Answer from the drawing. Dimensions are ordinates in mm from the lowest x, y and z of the part. A direction names the side the tool comes from. Round coordinates to 2 decimals unless told otherwise and drop trailing zeros. Write each loop counter-clockwise with the first axis right and the second up, starting at its lowest first coordinate (ties: lowest second). Pieces come first, ordered by that corner, then holes. Notation, with made-up numbers: (64.25, 26.5) -> (101.25, 26.5) arc R18 ccw to (101.25, 48.5) -> close; hole circle Ø1 at (45.25, -37.5). An arc over 180 degrees is marked (long way). Answer as a JSON object with one key per item and string values. Group by question number.
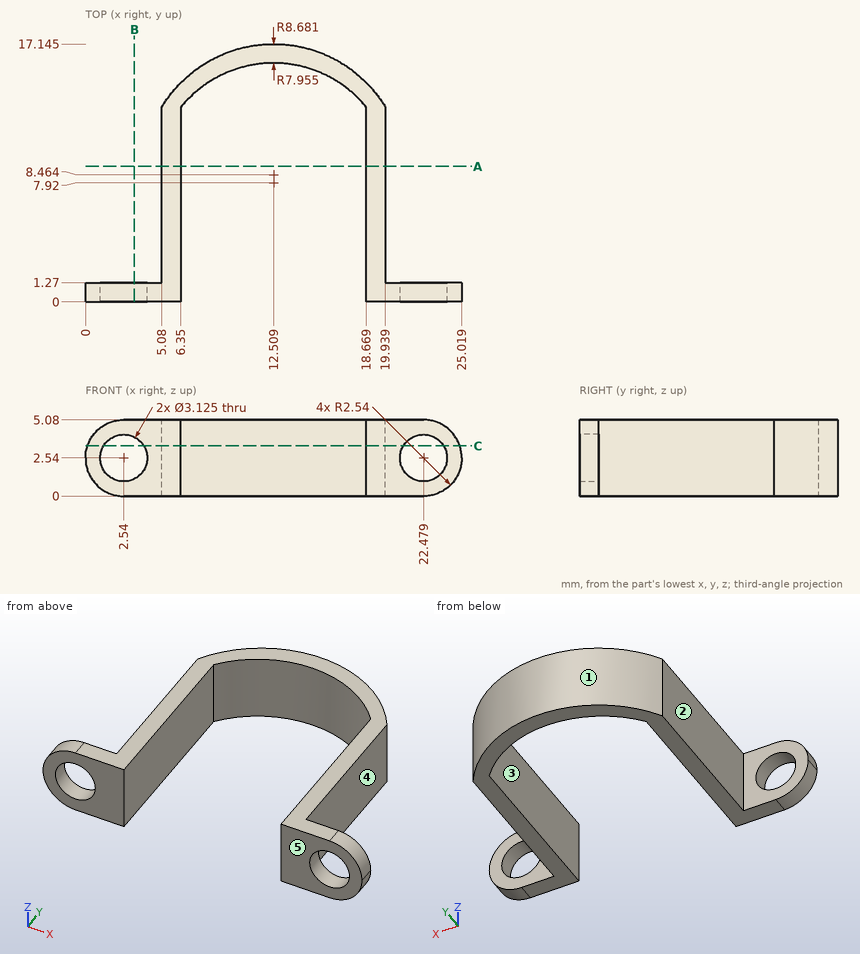
1) A cutting plane is placed at A-A on y = 9. Determine the outline of the cut face in (x, z).
2) A cutting plane is placed at B-B on x = 3.25. Determine the outline of the cut face in (y, z).
3) Each of these flat-tipped pins is pushed along its axis until it touches: P1, Ø3, axis at y = 10.5, z = 4.5, coming from the +X side; P2, Ø2.5, axis at x = 2.5, z = 3, coming from the +Y side; P3, Ø10, axis at x = 9, y = 5.5, coming from the +Z side; P4, Ø2, axis at x = 17, y = 8.5, coming from the +Z side. Where does it stop, or does it pass through?
4) Straight lines are drawn through the part: L1, parallel to X at y = 0.3, z = 2.54; L2, parallel to X at y = 4, z = 0.3; L3, parallel to Y at x = 24.25, z = 2.4. For each, find the intervals that lie inside material, in ascending order.
5) A tool of negligible diameter and unlimited length cuts with its end or side. For the marked faces 1, 2, 3, 4 and 5, from which of +Z, -Z, +X, -X, +Y, -Y can it reach the whole face along a straight path? Write none if from no direction.
6) A cutting plane is placed at C-C on z = 3.35. State how many separate pieces and enclosed holes the cut face has.
Established:
{
 "1": {"outline": "(5.08, 0) -> (6.35, 0) -> (6.35, 5.08) -> (5.08, 5.08) -> close; (18.67, 0) -> (19.94, 0) -> (19.94, 5.08) -> (18.67, 5.08) -> close"},
 "2": {"outline": "(0, 0) -> (1.27, 0) -> (1.27, 1.15) -> (0, 1.15) -> close; (0, 3.93) -> (1.27, 3.93) -> (1.27, 5.08) -> (0, 5.08) -> close"},
 "3": {"P1": "stops at x = 19.94", "P2": "stops at y = 1.27", "P3": "stops at z = 5.08", "P4": "passes through"},
 "4": {"L1": "x = 0 to 0.98, 4.1 to 6.35, 18.67 to 20.92, 24.04 to 25.02", "L2": "x = 5.08 to 6.35, 18.67 to 19.94", "L3": "y = 0 to 1.27"},
 "5": {"face 1": "+Z, -Z, +Y", "face 2": "+Z, -Z, -X, +Y", "face 3": "+Z, -Z, -Y", "face 4": "+Z, -Z, +X, +Y", "face 5": "+Z, -Z, +X, -X, -Y"},
 "6": {"separate pieces": "3", "enclosed holes": "0"}
}
